```python
from build123d import *


with BuildPart() as f1:
    # F0 (on Front) → F1 (revolve)
    with BuildSketch(Plane.XZ):
        with BuildLine():
            Line((0.914, 13.005), (0.914, 1.372))
            Line((0.914, 1.372), (1.143, 1.143))
            Line((1.143, 1.143), (1.143, -15.773))
            ThreePointArc((1.143, -15.773), (1.254592, -16.042408), (1.524, -16.154))
            Line((1.524, -16.154), (1.702, -16.154))
            ThreePointArc((1.702, -16.154), (2.151013, -15.968013), (2.337, -15.519))
            Line((2.337, -15.519), (2.337, 0))
            Line((2.337, 0), (2.946, 0))
            Line((2.946, 0), (2.946, 5.232))
            Line((2.946, 5.232), (1.955, 5.232))
            Line((1.955, 5.232), (1.955, 6.502))
            Line((1.955, 6.502), (2.946, 6.502))
            Line((2.946, 6.502), (2.946, 7.595))
            Line((2.946, 7.595), (1.955, 7.595))
            Line((1.955, 7.595), (1.955, 8.865))
            Line((1.955, 8.865), (2.946, 8.865))
            Line((2.946, 8.865), (2.946, 9.982))
            Line((2.946, 9.982), (1.955, 9.982))
            Line((1.955, 9.982), (1.955, 11.252))
            Line((1.955, 11.252), (2.946, 11.252))
            Line((2.946, 11.252), (2.946, 12.243))
            ThreePointArc((2.946, 12.243), (2.722815, 12.781815), (2.184, 13.005))
            Line((2.184, 13.005), (0.914, 13.005))
        make_face()
    revolve(axis=Axis((0, 0, 11.256295), (0, 0, 1)))


solid = f1.part
```
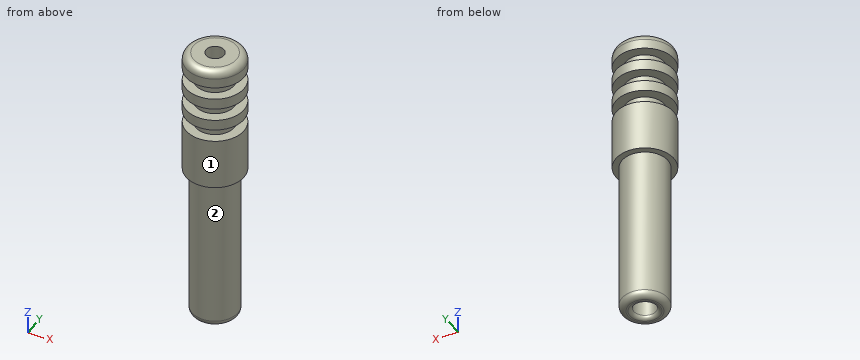
The listing builds one solid part. Answer for the finished solid, in the listing's coordinates (mm). Face numbers are marked on the shaded views. A direction names the side the tool comes from. Round coordinates to 2 decimals unless told otherwise and drop trailing zeros. Order: outer loops, then holes, each group sorted by start corner. A loop starts at its lowest first (then second) coordinate and runs counter-clockwise, first axis right, second up. Notation, with made-up numbers: (33.25, 14.5) -> (84.25, 14.5) arc R17 cw to (84.25, 36.5) -> close; hole circle Ø7 at (48.25, 48). An arc over 180 degrees is marked (long way). Answer as CSV lines item,"result".
Q1. Which of the six approach directions +Z, -Z, +X, -X, +Y, -Y give full straight-line access (tool end or side, diameter ignored) to the marked faces 1 and 2?
Computed values:
face 1,"+Z, -Z"
face 2,"-Z"
Q2. Given pin 1 (1 mm diameter, centred on y = 0.5, z = 6.5, fed in from -X), flat-ended and moving along its own axis, determine where the tip first touches the part or whether it passes through.
Computed values:
pin 1,"stops at x = -2.95"
Q3. Consider line 1 (Y direction, x = 0, z = 7.25); line 2 (Z direction, x = 1.45, y = 2.35) (3 decimals); line 3 (Y direction, x = 0, z = -7.5). Determine where each line is inside the solid, lowest interval first. Write a range as from..to.
Computed values:
line 1,"y = -2.95..-0.91, 0.91..2.95"
line 2,"z = 0..5.232, 6.502..7.595, 8.865..9.982, 11.252..12.74"
line 3,"y = -2.34..-1.14, 1.14..2.34"
Q4. A cutting plane is placed at A-A on z = -0.25. Determine the outline of the cut face in (x, y).
Computed values:
outline,"circle Ø4.67 at (0, 0); hole circle Ø2.29 at (0, 0)"
